```python
from build123d import *

# Parameters (mm, degrees)
CHAMFER_1_SIZE = 0.2


with BuildPart() as part:
    # 草图1 → 旋转1 (revolve)
    with BuildSketch(Plane.XY, mode=Mode.PRIVATE) as revolve_1_sk:
        Polygon((0, 3), (0, 29), (13.9, 29), (14, 28.9), (14.1, 29), (28, 29), (28, 13), (28, 10), (28, 3), align=None)
    revolve(revolve_1_sk.sketch.rotate(Axis((0, 0, 0), (1, 0, 0)), 90), axis=Axis((0, 0, 0), (1, 0, 0)))

    # 倒角1
    chamfer_1_edges = [part.edges().sort_by_distance(p)[0] for p in [
        (0, 0, -3),
        (28, 0, -29),
        (0, 0, -29),
    ]]
    chamfer(chamfer_1_edges, length=CHAMFER_1_SIZE)


solid = part.part
```
Can you work these out from the model? Positions are in its coordinate system, mm. Coordinates: 2 decimals unless noted, no trailing zeros. Loops run counter-clockwise (first coordinate to the right, second up) from the corner with the lowest first, then second, coordinate; pieces in that order, holes last. Notation, with made-up numbers: M -30,7.5 L 15,7.5 A30 cw 15,43.5 Z; hole C 29,-35.75 d2. An arc over 180 degrees is marked long. Put each result on its own line as item: value. Start each with the question number.
(1) Will these pins go through, and if not, where does the flat tip stop? pin 1 Ø5 at (y, z) = (0, 0) entering from +X; pin 2 Ø12 at (x, y) = (17.5, 20) entering from +Z; pin 3 Ø6 at (x, z) = (6, -17) entering from -Y; pin 4 Ø4 at (x, y) = (13.5, 10) entering from -Z.
(2) I need wall thicknesses on probe 1 along Y at (x, z) = (12.75, 0); probe 2 along Z at (x, y) = (6.75, -0.5); probe 3 along Y at (x, z) = (2.5, 2). Which ranges of each line are inside material? Lowest first, please.
(3) Imagine slicing it at C-C on x = 4.25. List the corners of the cut face in (y, z) for me.
(4) Imagine slicing it at A-A on y = 0. List the corners of the cut face in (x, z) for me, and give its area (3 significant figures).
Worked answers:
1. pin 1: passes through
1. pin 2: stops at z = 25.4
1. pin 3: stops at y = -25.4
1. pin 4: stops at z = -27.87
2. probe 1: y = -29 to -3, 3 to 29
2. probe 2: z = -29 to -2.96, 2.96 to 29
2. probe 3: y = -28.93 to -2.24, 2.24 to 28.93
3. outline: C 0,0 d58; hole C 0,0 d6
4. outline: M 0,-28.8 L 0.2,-29 L 13.9,-29 L 14,-28.9 L 14.1,-29 L 27.8,-29 L 28,-28.8 L 28,-3 L 0.2,-3 L 0,-3.2 Z; M 0,3.2 L 0.2,3 L 28,3 L 28,28.8 L 27.8,29 L 14.1,29 L 14,28.9 L 13.9,29 L 0.2,29 L 0,28.8 Z
4. area: 1,460 mm2
